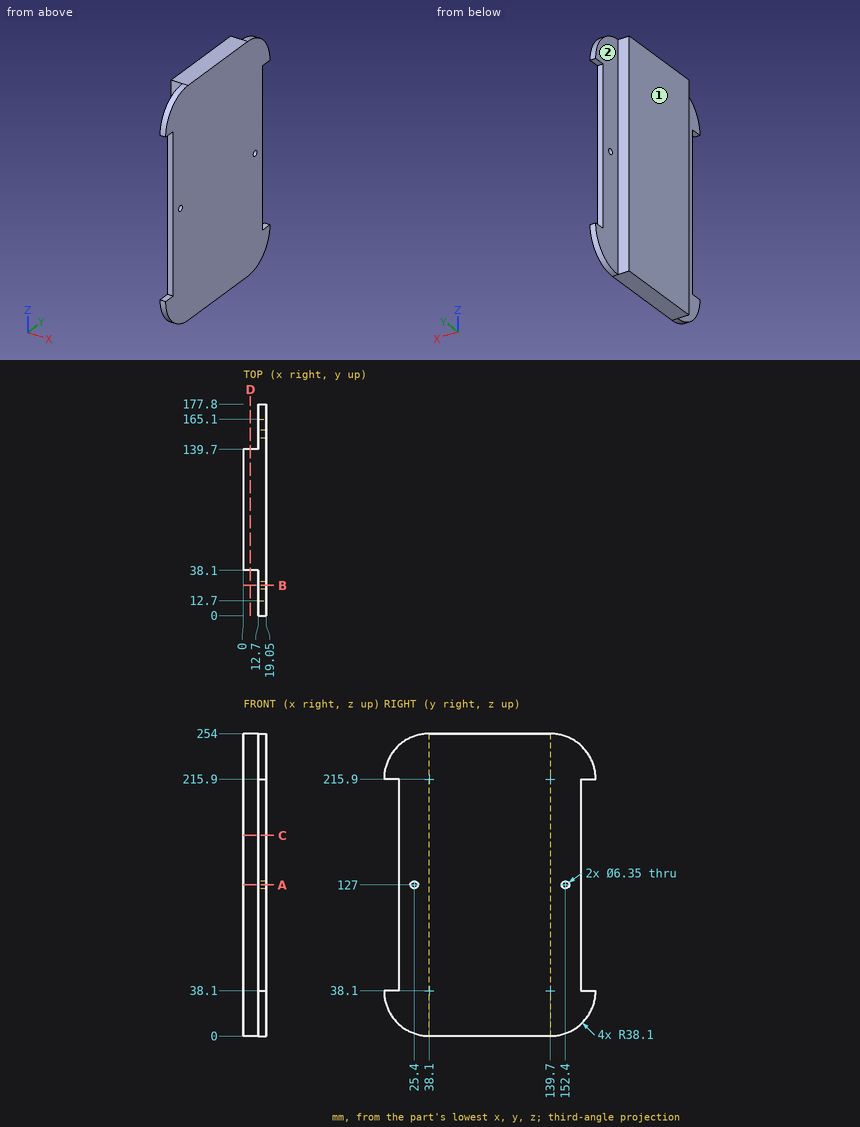
The figure shows three views and two pictorial views of one solid part (mm, origin at its lowest corner). Answer the questions. A direction names the side the tool comes from. Give positions to 0.01 mm unless a question says otherwise; leave off trailing zeros. Loops run counter-clockwise (first coordinate to the right, second up) from the corner with the lowest first, then second, coordinate; pieces in that order, holes last. Notation, with made-up numbers: (85.5, 60) -> (117.5, 60) arc R15 cw to (117.5, 83) -> close; hole circle Ø10 at (-20.75, 80.5). An arc over 180 degrees is marked (long way). Put each result on its own line as item: value. Start each with the question number.
Item 1: Each of these flat-tipped pins is pushed along its axis until it touches: P1, Ø2, axis at x = 4.5, z = 114.5, coming from the -Y side; P2, Ø6, axis at y = 158, z = 86, coming from the -X side; P3, Ø3, axis at x = 12, y = 150.5, coming from the +Z side; P4, Ø10, axis at y = 90.5, z = 98, coming from the -X side. Where does it stop, or does it pass through?
Item 2: Find the intervals of material crossed by L1, parallel to Y at x = 14.5, z = 127 (3 decimals); L2, parallel to X at y = 32, z = 47; L3, parallel to Y at x = 16, z = 45, in increasing order. Write a range as [from, to].
Item 3: Which of the six approach directions +Z, -Z, +X, -X, +Y, -Y give full straight-line access (tool end or side, diameter ignored) to the marked faces 1 and 2?
Item 4: The part is cut by section B-B (y = 25.4). Give the vertices of the cut face in (x, z) (3 decimals), then the cut area to 3 significant figures.
Item 5: The part is cut by section C-C (z = 168.5). Give the vertices of the cut face in (x, y).
Item 6: The part is cut by section A-A (z = 127). Give the vertices of the cut face in (x, y) (3 decimals), then the cut area to 3 significant figures.
Item 7: The part is cut by section D-D (x = 6). Give the vertices of the cut face in (y, z), then the cut area to 3 significant figures.
Answers below:
1. P1: y = 38.1
1. P2: x = 12.7
1. P3: z = 252.8
1. P4: x = 0
2. L1: [12.7, 22.225], [28.575, 149.225], [155.575, 165.1]
2. L2: [12.7, 19.05]
2. L3: [12.7, 165.1]
3. face 1: +Z, -Z, -X, +Y, -Y
3. face 2: +Z, -Z, -X, +Y
4. outline: (12.7, 2.179) -> (19.05, 2.179) -> (19.05, 123.825) -> (12.7, 123.825) -> close; (12.7, 130.175) -> (19.05, 130.175) -> (19.05, 251.821) -> (12.7, 251.821) -> close
4. area: 1,540 mm2
5. outline: (0, 38.1) -> (12.7, 38.1) -> (12.7, 12.7) -> (19.05, 12.7) -> (19.05, 165.1) -> (12.7, 165.1) -> (12.7, 139.7) -> (0, 139.7) -> close
6. outline: (0, 38.1) -> (12.7, 38.1) -> (12.7, 28.575) -> (19.05, 28.575) -> (19.05, 149.225) -> (12.7, 149.225) -> (12.7, 139.7) -> (0, 139.7) -> close; (12.7, 12.7) -> (19.05, 12.7) -> (19.05, 22.225) -> (12.7, 22.225) -> close; (12.7, 155.575) -> (19.05, 155.575) -> (19.05, 165.1) -> (12.7, 165.1) -> close
6. area: 2,180 mm2
7. outline: (38.1, 0) -> (139.7, 0) -> (139.7, 254) -> (38.1, 254) -> close
7. area: 25,800 mm2
